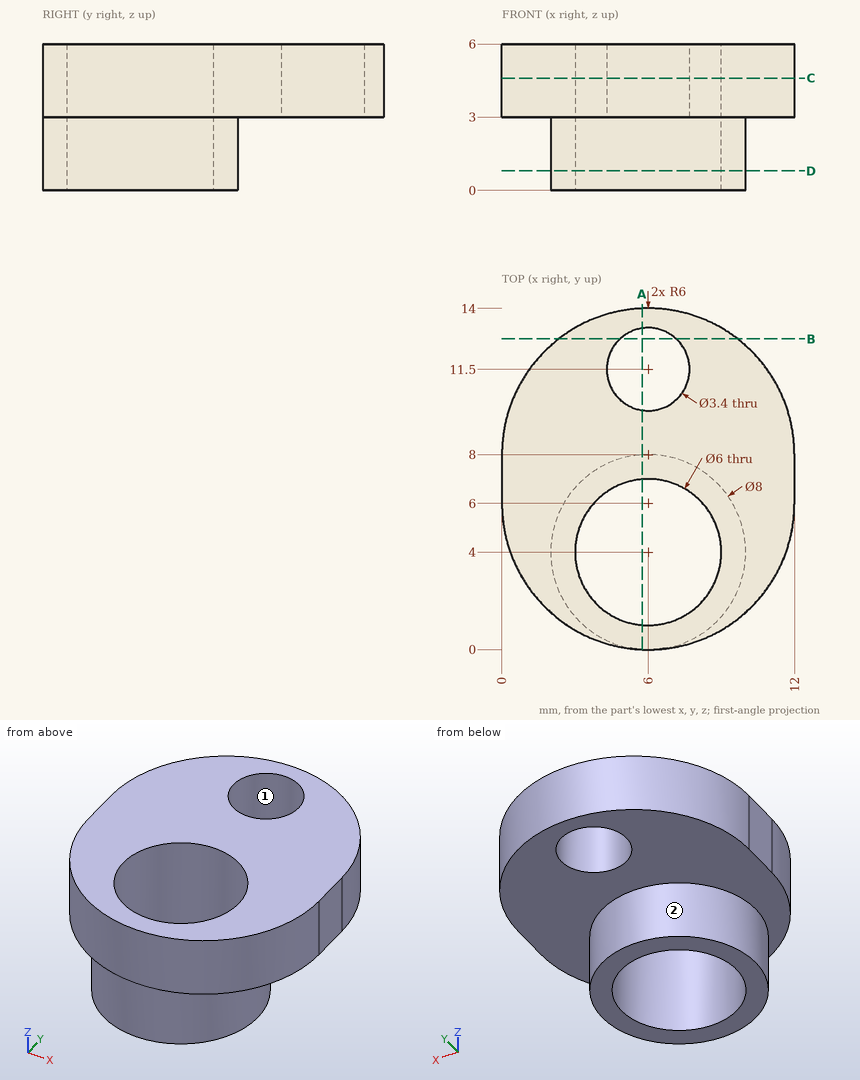
Print and shaded views of the part. All mm, measured from the part's lowest x, y and z. A direction names the side the tool comes from. Give positions to 0.01 mm unless a question says otherwise; leave off trailing zeros. Write each loop counter-clockwise with the first axis right and the second up, starting at its lowest first coordinate (ties: lowest second). Pieces come first, ordered by that corner, then holes. Notation, with made-up numbers: (46, -2.75) - (59, -2.75) arc R22 cw to (59, 14.25) - close; hole circle Ø9 at (7.5, 60.5). An arc over 180 degrees is marked (long way). One line per question, with ' | ' between items. Start each with the question number.
(1) Wall check: line 1 along Y through (x, z) = (6, 4.05); line 2 along Y through (x, z) = (6, 2.6); line 3 along X through (y, z) = (11.75, 4.85). Give the ranges that are in metal, low to high. Write a range as from..to.
(2) Slice it at A-A on x = 5.75. Give the number of separate pieces and of enclosed holes in the cut face, plus the area to 3 significant figures.
(3) Slice it at B-B on y = 12.75. Write the cut outline in (x, z), plus the area to 3 significant figures.
(4) Pin check, flat tips, straight feed: P1, Ø1, axis at x = 5, z = 4, coming from the +Y side; P2, Ø4, axis at x = 6, y = 11.5, coming from the +Z side. Stop position of each tip, or through.
(5) 3-axis set-ups, long thin cutter, end or side, ignore diameter. For the marked faces 1 and 2: which of +Z, -Z, +X, -X, +Y, -Y reach the whole face in a straight line?
(6) Slice it at D-D on z = 0.8. Write the cut outline in (x, y), plus the area to 3 significant figures.
(7) Slice it at C-C on z = 4.6. Write the cut outline in (x, y), plus the area to 3 significant figures.
Results below:
1) line 1: 0..1, 7..9.8, 13.2..14 | line 2: 0..1, 7..8 | line 3: 1.32..4.32, 7.68..10.68
2) separate pieces: 3 | enclosed holes: 0 | area: 20.0 mm^2
3) outline: (2.33, 3) - (4.85, 3) - (4.85, 6) - (2.33, 6) - close; (7.15, 3) - (9.67, 3) - (9.67, 6) - (7.15, 6) - close | area: 15.1 mm^2
4) P1: y = 13.98 | P2: z = 6
5) face 1: +Z, -Z | face 2: -Z
6) outline: circle Ø8 at (6, 4); hole circle Ø6 at (6, 4) | area: 22.0 mm^2
7) outline: (0, 6) arc R6 ccw to (12, 6) - (12, 8) arc R6 ccw to (0, 8) - close; hole circle Ø6 at (6, 4); hole circle Ø3.4 at (6, 11.5) | area: 99.7 mm^2
